from build123d import *

# Parameters (mm, degrees)
SKETCH1_R           = 1.5
SKETCH1_R_2         = 1.55
BOSS_EXTRUDE1_DEPTH = 6


with BuildPart() as part:
    # Sketch1 → Boss-Extrude1 (new body)
    with BuildSketch(Plane(origin=(0, 0, 0), x_dir=(1, 0, 0), z_dir=(0, 1, 0))):
        with BuildLine():
            Line((-10.054576391, 17.239228809), (-18.654572416, 16.912740777))
            ThreePointArc((-18.654572416, 16.912740777), (-25.479153077, 13.855584783), (-28.275208275, 6.919939226))
            Line((-28.275208275, 6.919939226), (-28.275208275, 0))
            Line((-28.275208275, 0), (-49.137604137, 0))
            Line((-49.137604137, 0), (-70, 0))
            Line((-70, 0), (-51.187164382, -9.017581558))
            ThreePointArc((-51.187164382, -9.017581558), (-49.081079033, -9.751302876), (-46.864755002, -10))
            Line((-46.864755002, -10), (0, -10))
            Line((0, -10), (15, -10))
            Line((15, -10), (1.155446716, -0.770297811))
            add(Edge.make_bspline(
                [(1.155446716, -0.770297811), (2.094509546, -0.481388498), (3.042693974, -0.224622561), (4, 0)],
                knots=[0.265250857, 0.265250857, 0.265250857, 0.265250857, 1, 1, 1, 1], degree=3))
            Line((4, 0), (8, 0))
            ThreePointArc((8, 0), (11, 3), (8, 6))
            Line((8, 6), (4, 6))
            add(Edge.make_bspline(
                [(0.141983447, 7.095761644), (2.045647207, 6.458569901), (4, 6)],
                knots=[0, 0, 0, 1, 1, 1], degree=2))
            ThreePointArc((0.141983447, 7.095761644), (-2.383666412, 14.242578452), (-9.33430338, 17.266573068))
            Line((-9.33430338, 17.266573068), (-10.054576391, 17.239228809))
        make_face()
        with Locations((-35.063841459, -5)):
            Circle(SKETCH1_R, mode=Mode.SUBTRACT)
        with Locations((8, 3)):
            Circle(SKETCH1_R, mode=Mode.SUBTRACT)
        with Locations((-9.33430338, 7.766573068)):
            Circle(SKETCH1_R_2, mode=Mode.SUBTRACT)
    extrude(amount=BOSS_EXTRUDE1_DEPTH)


solid = part.part
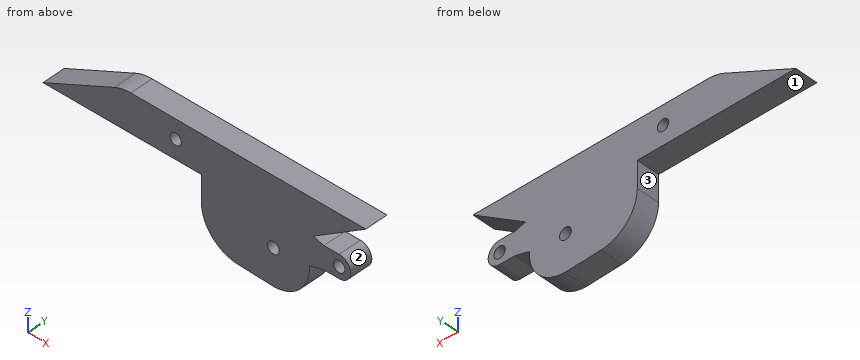
Geometry: final body of the model. Coordinates: model frame, mm. Face numbers are marked on the shaded views. Round coordinates to 2 decimals unless told otherwise and drop trailing zeros. Loops run counter-clockwise (first coordinate to the right, second up) from the corner with the lowest first, then second, coordinate; pieces in that order, holes last. Notation, with made-up numbers: M 15,54 L 53,54 A18 cw 53,83 Z; hole C -25.5,67.5 d4. An arc over 180 degrees is marked long. Put each result on its own line as item: value. Start each with the question number.
(1) Draft query along Z for the marked faces 1, 2 and 3. Return one class per face: +Z half, -Z half, draft (parallel to the pull), parting line (faces both ways), or undercut.
(2) Material intervals for line 1 along X through (y, z) = (1.95, -3); line 2 along X through (y, z) = (2.75, 5); line 3 along Z through (x, y) = (-42, 1.75), sorted ascending. Write a range as [from, to].
(3) Section query C-C (x = -42.5). Return loops of the section in (y, z).
(4) Section query B-B (y = 2). State how many separate pieces and enclosed holes the cut face has, then the cut area to 3 significant figures.
(5) Contact query for flat-ended pins moving along their axis: pin 1 Ø3 at (y, z) = (4.5, -12) entering from +X; pin 2 Ø2 at (x, y) = (5.5, 3) entering from -Z; pin 3 Ø3 at (y, z) = (3, -2.5) entering from -X. Output: stop coordinate, or through.
(6) Section query D-D (z = 5). Return loops of the section in (x, y), then the cut area to 3 significant figures.
(7) Section query A-A (z = -3). Return loops of the section in (x, y).
Findings below:
1. face 1: -Z half
1. face 2: undercut
1. face 3: draft
2. line 1: x = [-28.28, 6.5], [9.5, 11]
2. line 2: x = [-59.57, -36.56], [-33.56, 7.5]
2. line 3: z = [0, 10]
3. outline: M 0,0 L 6,0 L 6,10 L 0,10 Z
4. separate pieces: 1
4. enclosed holes: 3
4. area: 1,160 mm2
5. pin 1: stops at x = -0.24
5. pin 2: stops at z = -6
5. pin 3: stops at x = -28.28
6. outline: M -59.57,0 L -36.56,0 L -36.56,6 L -59.57,6 Z; M -33.56,0 L 7.5,0 L 7.5,6 L -33.56,6 Z
6. area: 384 mm2
7. outline: M -28.28,0 L 6.5,0 L 6.5,6 L -28.28,6 Z; M 9.5,0 L 11,0 L 11,6 L 9.5,6 Z
